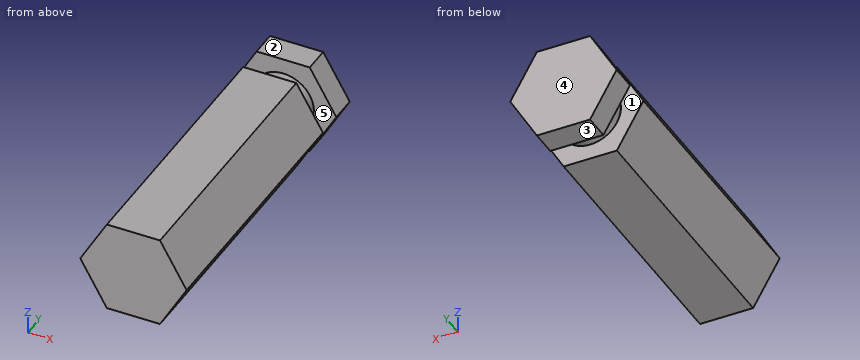
```python
from build123d import *

# Parameters (mm, degrees)
BOSS_EXTRUDE1_DEPTH = 61
SKETCH2_R           = 7
BOSS_EXTRUDE2_DEPTH = 6
BOSS_EXTRUDE3_DEPTH = 6


with BuildPart() as part:
    # Sketch1 → Boss-Extrude1 (new body)
    with BuildSketch(Plane(origin=(0, 0, 0), x_dir=(1, 0, 0), z_dir=(0, 1, 0))):
        Polygon((-12.124355653, 0), (-6.062177826, -10.5), (6.062177826, -10.5), (12.124355653, 0), (6.062177826, 10.5), (-6.062177826, 10.5), align=None)
    extrude(amount=BOSS_EXTRUDE1_DEPTH)

    # Sketch2 → Boss-Extrude2 (add)
    with BuildSketch(Plane(origin=(0, 61, 0), x_dir=(1, 0, 0), z_dir=(0, 1, 0))):
        with Locations(Location((0, 0, 0), (0, 0, 270))):
            Circle(SKETCH2_R)
    extrude(amount=BOSS_EXTRUDE2_DEPTH)

    # Sketch3 → Boss-Extrude3 (add)
    with BuildSketch(Plane(origin=(0, 67, 0), x_dir=(1, 0, 0), z_dir=(0, 1, 0))):
        Polygon((-12.124355653, 0), (-6.062177826, -10.5), (6.062177826, -10.5), (12.124355653, 0), (6.062177826, 10.5), (-6.062177826, 10.5), align=None)
    extrude(amount=BOSS_EXTRUDE3_DEPTH)


solid = part.part
```
Can you work these out from the model? Positions are in its coordinate system, mm. Face numbers are marked on the shaded views. A direction names the side the tool comes from. Coordinates: 2 decimals unless noted, no trailing zeros. Write each loop counter-clockwise with the first axis right and the second up, starting at its lowest first coordinate (ties: lowest second). Pieces come first, ordered by that corner, then holes. Notation, with made-up numbers: M 11,-30.75 L 53,-30.75 A17 cw 53,-10.75 Z; hole C 33.5,44.5 d9. An arc over 180 degrees is marked long. Write item = value, one per line. Start each with the question number.
Q1. Thinking about a two-plate mould opening in Y: for the marked faces 3, 4 and 5, which applies, released by +Y, released by -Y, zero draft, split by the parting line, or undercut?
Q2. If we section it at B-B, the plane x = 0: Write out the boundary of the cut face in (y, z).
Q3. I'm going to push flat-ended pins straight in: pin 1 (8 mm diameter, centred on x = 4, z = -3, fed in from -Y); pin 2 (12 mm diameter, centred on y = 31, z = 8, fed in from -X); pin 3 (4 mm diameter, centred on y = 26, z = 3, fed in from -X); pin 4 (1.5 mm diameter, centred on x = -7.5, y = 53, fed in from +Z). Where does each tip first touch, or does it pass through?
Q4. If we section it at A-A, the plane y = 52: Write out the boundary of the cut face in (x, z).
Q5. If we section it at C-C, the plane z = -2: Write out the boundary of the cut face in (x, y), then the cut area to 3 significant figures.
Q6. On a 3-axis mill with a long thin cutter (end or side, diameter ignored), from which of +Z, -Z, +X, -X, +Y, -Y can I reach the whole of each face in a straight line? I mean the marked faces 1 and 2. Say none if no direction works.
Q7. If I drill on L1, parallel to Y at x = 11.25, z = -0.5; L2, parallel to X at y = 8, z = 5.25; L3, parallel to X at y = 49, z = -8.5, over which ranges is the centre line in solid material (lowest first)? Write a range as [from, to].
Q8. If we section it at D-D, the plane z = 7.75: Write out the boundary of the cut face in (x, y).
Check sheet entries:
q1.face_3 = zero draft
q1.face_4 = released by +Y
q1.face_5 = undercut
q2.outline = M 0,-10.5 L 61,-10.5 L 61,-7 L 67,-7 L 67,-10.5 L 73,-10.5 L 73,10.5 L 67,10.5 L 67,7 L 61,7 L 61,10.5 L 0,10.5 Z
q3.pin_1 = 0
q3.pin_2 = -10.97
q3.pin_3 = -11.55
q3.pin_4 = 9.31
q4.outline = M -12.12,0 L -6.06,-10.5 L 6.06,-10.5 L 12.12,0 L 6.06,10.5 L -6.06,10.5 Z
q5.outline = M -10.97,0 L 10.97,0 L 10.97,61 L 6.71,61 L 6.71,67 L 10.97,67 L 10.97,73 L -10.97,73 L -10.97,67 L -6.71,67 L -6.71,61 L -10.97,61 Z
q5.area = 1,550 mm²
q6.face_1 = none
q6.face_2 = +Z, +X, -X, +Y, -Y
q7.L1 = [0, 61], [67, 73]
q7.L2 = [-9.09, 9.09]
q7.L3 = [-7.22, 7.22]
q8.outline = M -7.65,0 L 7.65,0 L 7.65,61 L -7.65,61 Z; M -7.65,67 L 7.65,67 L 7.65,73 L -7.65,73 Z
